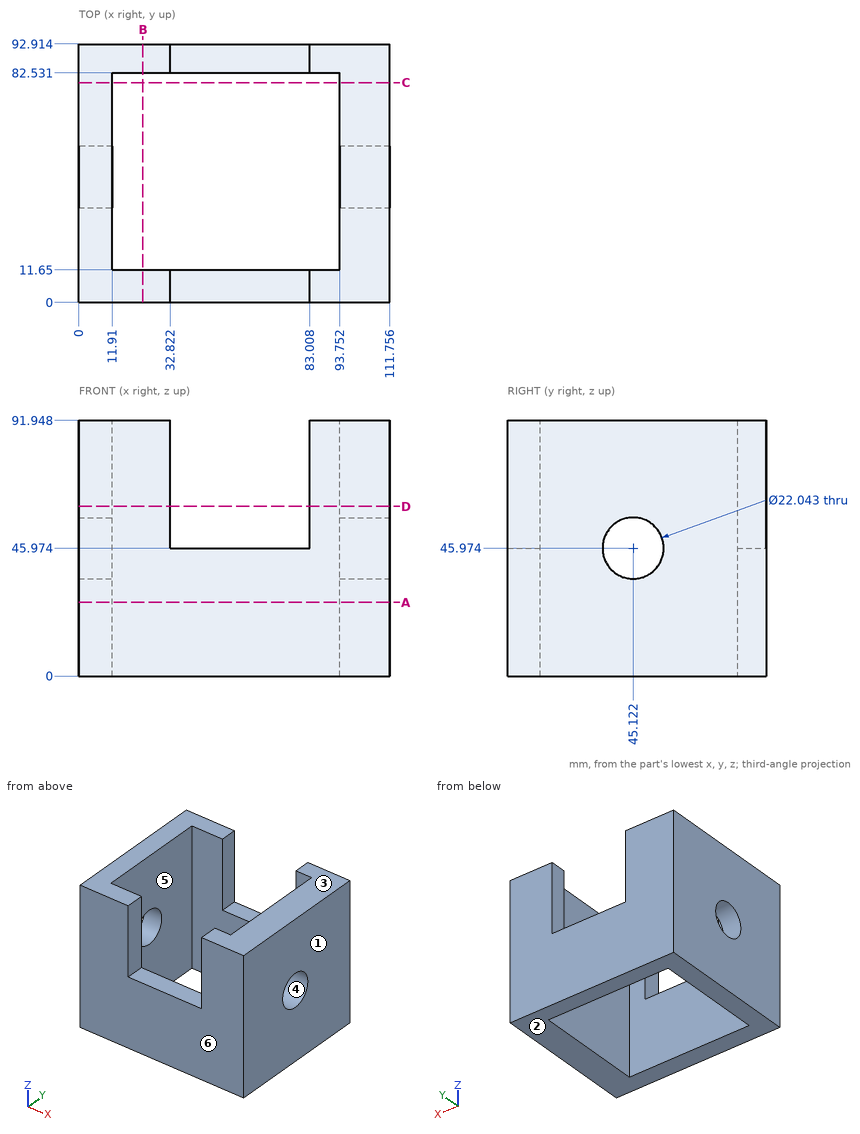
Check sheet for the drawn part. Datum: minimum x, y, z corner. Units: mm. A direction names the side the tool comes from. Coordinates: 2 decimals unless noted, no trailing zeros. Loops run counter-clockwise (first coordinate to the right, second up) from the corner with the lowest first, then second, coordinate; pieces in that order, holes last. Notation, with made-up numbers: (13, 63) -> (31, 63) arc R21 cw to (31, 92) -> close; hole circle Ø4 at (-16.75, 82.25). An arc over 180 degrees is marked (long way). Answer as CSV lines item,"result".
1) Depth check by flat-ended pin: pin 1 (5 mm diameter, centred on y = 59, z = 37.5, fed in from -X); pin 2 (6 mm diameter, centred on x = 62.5, y = 7, fed in from +Z); pin 3 (13 mm diameter, centred on y = 45.12, z = 45.97, fed in from +X). Enter the tip coordinate at first touch or a pass-through.
Found:
pin 1,"stops at x = 0"
pin 2,"stops at z = 45.97"
pin 3,"passes through"
2) Cross-section at C-C, the plane y = 79. Record the cut outline in (x, z), then the cut area to 3 significant figures.
Found:
outline,"(0, 0) -> (11.91, 0) -> (11.91, 91.95) -> (0, 91.95) -> close; (93.75, 0) -> (111.76, 0) -> (111.76, 91.95) -> (93.75, 91.95) -> close"
area,"2,750 mm2"
3) Cross-section at A-A, the plane z = 26.5. Record the cut outline in (x, y).
Found:
outline,"(0, 0) -> (111.76, 0) -> (111.76, 92.91) -> (0, 92.91) -> close; hole (11.91, 11.65) -> (93.75, 11.65) -> (93.75, 82.53) -> (11.91, 82.53) -> close"
4) Cross-section at B-B, the plane x = 23. Record the cut outline in (y, z).
Found:
outline,"(0, 0) -> (11.65, 0) -> (11.65, 91.95) -> (0, 91.95) -> close; (82.53, 0) -> (92.91, 0) -> (92.91, 91.95) -> (82.53, 91.95) -> close"
5) Thickness scan on L1, parallel to X at y = 88.5, z = 58; L2, parallel to Y at x = 28, z = 5; L3, parallel to X at y = 60, z = 48. Record the ranges inside material, lowest first. Write a range as from..to.
Found:
L1,"x = 0..32.82, 83.01..111.76"
L2,"y = 0..11.65, 82.53..92.91"
L3,"x = 0..11.91, 93.75..111.76"
6) Cross-section at D-D, the plane z = 61. Record the cut outline in (x, y), then the cut area to 3 significant figures.
Found:
outline,"(0, 0) -> (32.82, 0) -> (32.82, 11.65) -> (11.91, 11.65) -> (11.91, 82.53) -> (32.82, 82.53) -> (32.82, 92.91) -> (0, 92.91) -> close; (83.01, 0) -> (111.76, 0) -> (111.76, 92.91) -> (83.01, 92.91) -> (83.01, 82.53) -> (93.75, 82.53) -> (93.75, 11.65) -> (83.01, 11.65) -> close"
area,"3,480 mm2"
7) Tool access check on the marked faces 5 and 6. Record the directions out of +Z, -Z, +X, -X, +Y, -Y that give a thin tool (end or side, any length) a straight path to the whole face; none if there is none.
Found:
face 5,"+Z, -Z"
face 6,"+Z, -Z, +X, -X, -Y"
8) Release check for a two-part mould opening along Z. For the marked faces 1, 2, 3 and 4 record: +Z half, -Z half, draft (parallel to the pull), parting line (faces both ways), or undercut.
Found:
face 1,"draft"
face 2,"-Z half"
face 3,"+Z half"
face 4,"undercut"
